from build123d import *

# Parameters (mm, degrees)
SKETCH1_W           = 113.65
SKETCH1_H           = 36.2
SKETCH1_W_2         = 109.65
SKETCH1_H_2         = 32.2
SKETCH1_W_3         = 107.65
SKETCH1_H_3         = 30.2
BOSS_EXTRUDE1_DEPTH = 2
BOSS_EXTRUDE2_DEPTH = 11.65
SKETCH3_W           = 38
SKETCH3_H           = 8
SKETCH3_R           = 1.7
BOSS_EXTRUDE3_DEPTH = 2
SKETCH4_W           = 22
SKETCH4_H           = 8
SKETCH4_R           = 1.6
BOSS_EXTRUDE4_DEPTH = 11.65
SKETCH5_W           = 14
SKETCH5_H           = 2
CUT_EXTRUDE1_DEPTH  = 11.65


with BuildPart() as part:
    # Sketch1 → Boss-Extrude1 (new body)
    # profile 1 of 3: a face of its own
    with BuildSketch(Plane(origin=(0, 0, 0), x_dir=(1, 0, 0), z_dir=(0, 1, 0))):
        with Locations((53.825, 15.1)):
            Rectangle(SKETCH1_W, SKETCH1_H)
        with Locations((53.825, 15.1)):
            Rectangle(SKETCH1_W_2, SKETCH1_H_2, mode=Mode.SUBTRACT)
    # profile 2 of 3: a face of its own
    with BuildSketch(Plane(origin=(0, 0, 0), x_dir=(1, 0, 0), z_dir=(0, 1, 0))):
        with Locations((53.825, 15.1)):
            Rectangle(SKETCH1_W_2, SKETCH1_H_2)
        with Locations((53.825, 15.1)):
            Rectangle(SKETCH1_W_3, SKETCH1_H_3, mode=Mode.SUBTRACT)
    # profile 3 of 3: a face of its own
    with BuildSketch(Plane(origin=(0, 0, 0), x_dir=(1, 0, 0), z_dir=(0, 1, 0))):
        with Locations((53.825, 15.1)):
            Rectangle(SKETCH1_W_3, SKETCH1_H_3)
    extrude(amount=BOSS_EXTRUDE1_DEPTH)

    # Sketch2 → Boss-Extrude2 (add)
    with BuildSketch(Plane(origin=(0, 2, 0), x_dir=(1, 0, 0), z_dir=(0, 1, 0))):
        Polygon((15, -1), (15, -3), (-3, -3), (-3, 10.1), (-1, 10.1), (-1, -1), align=None)
        Polygon((-1, 20.1), (-3, 20.1), (-3, 33.2), (110.65, 33.2), (110.65, 23.1), (108.65, 23.1), (108.65, 31.2), (-1, 31.2), align=None)
        Polygon((108.65, -1), (108.65, 7.1), (110.65, 7.1), (110.65, -3), (87.65, -3), (87.65, -1), align=None)
    extrude(amount=BOSS_EXTRUDE2_DEPTH)

    # Sketch3 → Boss-Extrude3 (add)
    with BuildSketch(Plane.XZ):
        with Locations((53.825, -37.2)):
            Rectangle(SKETCH3_W, SKETCH3_H)
        with Locations(Location((68.825, -37.2, 0), (0, 0, 90))):
            Circle(SKETCH3_R, mode=Mode.SUBTRACT)
        with Locations(Location((38.825, -37.2, 0), (0, 0, 90))):
            Circle(SKETCH3_R, mode=Mode.SUBTRACT)
    extrude(amount=-BOSS_EXTRUDE3_DEPTH)

    # Sketch4 → Boss-Extrude4 (add)
    with BuildSketch(Plane(origin=(0, 2, 0), x_dir=(1, 0, 0), z_dir=(0, 1, 0))):
        with Locations((53.825, 37.2)):
            Rectangle(SKETCH4_W, SKETCH4_H)
        with Locations(Location((46.825, 37.2, 0), (0, 0, 270))):
            Circle(SKETCH4_R, mode=Mode.SUBTRACT)
        with Locations(Location((60.825, 37.2, 0), (0, 0, 90))):
            Circle(SKETCH4_R, mode=Mode.SUBTRACT)
    extrude(amount=BOSS_EXTRUDE4_DEPTH)

    # Sketch5 → Cut-Extrude1 (cut)
    with BuildSketch(Plane(origin=(0, 13.65, 0), x_dir=(1, 0, 0), z_dir=(0, 1, 0))):
        with Locations((74.825, 32.2)):
            Rectangle(SKETCH5_W, SKETCH5_H)
    extrude(amount=-CUT_EXTRUDE1_DEPTH, mode=Mode.SUBTRACT)


solid = part.part
Source: CAD feature listing. Evaluate the final solid. Frame: model axes, mm. A direction names the side the tool comes from. Give positions to 0.01 mm unless a question says otherwise; leave off trailing zeros. Write each loop counter-clockwise with the first axis right and the second up, starting at its lowest first coordinate (ties: lowest second). Pieces come first, ordered by that corner, then holes. Notation, with made-up numbers: (-22, 44.5) -> (-12, 44.5) arc R20 ccw to (-12, 81.5) -> close; hole circle Ø5 at (16, 80). An arc over 180 degrees is marked (long way). Write item = value, one per line.
Q1. Reachability of faces 1 (the face through (41, 2, -37)), 2 (the face through (95, 8, -31.2)), 3 (the face through (110, 8, -23.1)), 4 (the face through (96, 7, -33.2)) from +Z, -Z, +X, -X, +Y, -Y: full face, straight path, thin tool, end or side. Return the list, or none.
Here are the results:
face_1 = -Z, -X, +Y
face_2 = +Y
face_3 = +X, +Y
face_4 = -Z, +X, +Y, -Y
Q2. Cut plane A-A on z = -37.2. Return loops of the section in (x, y) (3 decimals).
Here are the results:
outline = (34.825, 0) -> (37.125, 0) -> (37.125, 2) -> (34.825, 2) -> close; (40.525, 0) -> (67.125, 0) -> (67.125, 2) -> (64.825, 2) -> (64.825, 13.65) -> (62.425, 13.65) -> (62.425, 2) -> (59.225, 2) -> (59.225, 13.65) -> (48.425, 13.65) -> (48.425, 2) -> (45.225, 2) -> (45.225, 13.65) -> (42.825, 13.65) -> (42.825, 2) -> (40.525, 2) -> close; (70.525, 0) -> (72.825, 0) -> (72.825, 2) -> (70.525, 2) -> close
Q3. First-contact query: pin 1 (7 mm diameter, centred on x = 17, y = 3.5, fed in from -Z); pin 2 (2.5 mm diameter, centred on x = 60.825, z = -37.2, fed in from +Y); pin 3 (6 mm diameter, centred on x = 48, y = 6.5, fed in from +Z). Flat tips, straight axial feed; report the tip coordinate or a pass-through.
Here are the results:
pin_1 = -33.2
pin_2 = 2
pin_3 = -31.2
Q4. Cut plane B-B on y = 6.5. State how many separate pieces and enclosed holes the cut face has, then the cut area to 3 significant figures.
Here are the results:
separate_pieces = 4
enclosed_holes = 2
area = 518 mm²
Q5. Cut plane C-C on x = 57.5. Return loops of the section in (y, z), then the cut area to 3 significant figures.
Here are the results:
outline = (0, -41.2) -> (13.65, -41.2) -> (13.65, -31.2) -> (2, -31.2) -> (2, 3) -> (0, 3) -> close
area = 205 mm²
Q6. Line query: line 1 (X direction, y = 1.4, z = -37.2) (3 decimals); line 2 (X direction, y = 7.25, z = -37.2) (3 decimals); line 3 (Z direction, x = 12.5, y = 6.25). Output: solid intervals per line, ascending. Write a range as from..to.
Here are the results:
line_1 = 34.825..37.125, 40.525..67.125, 70.525..72.825
line_2 = 42.825..45.225, 48.425..59.225, 62.425..64.825
line_3 = -33.2..-31.2, 1..3
